Print and shaded views of the part. All mm, measured from the part's lowest x, y and z. A direction names the side the tool comes from. Give positions to 0.01 mm unless a question says otherwise; leave off trailing zeros. Loops run counter-clockwise (first coordinate to the right, second up) from the corner with the lowest first, then second, coordinate; pieces in that order, holes last. Notation, with made-up numbers: M 46.5,81 L 90.5,81 A33 cw 90.5,117 Z; hole C 48.25,39 d6. An arc over 180 degrees is marked long. Answer in a Markdown table with one row per item.
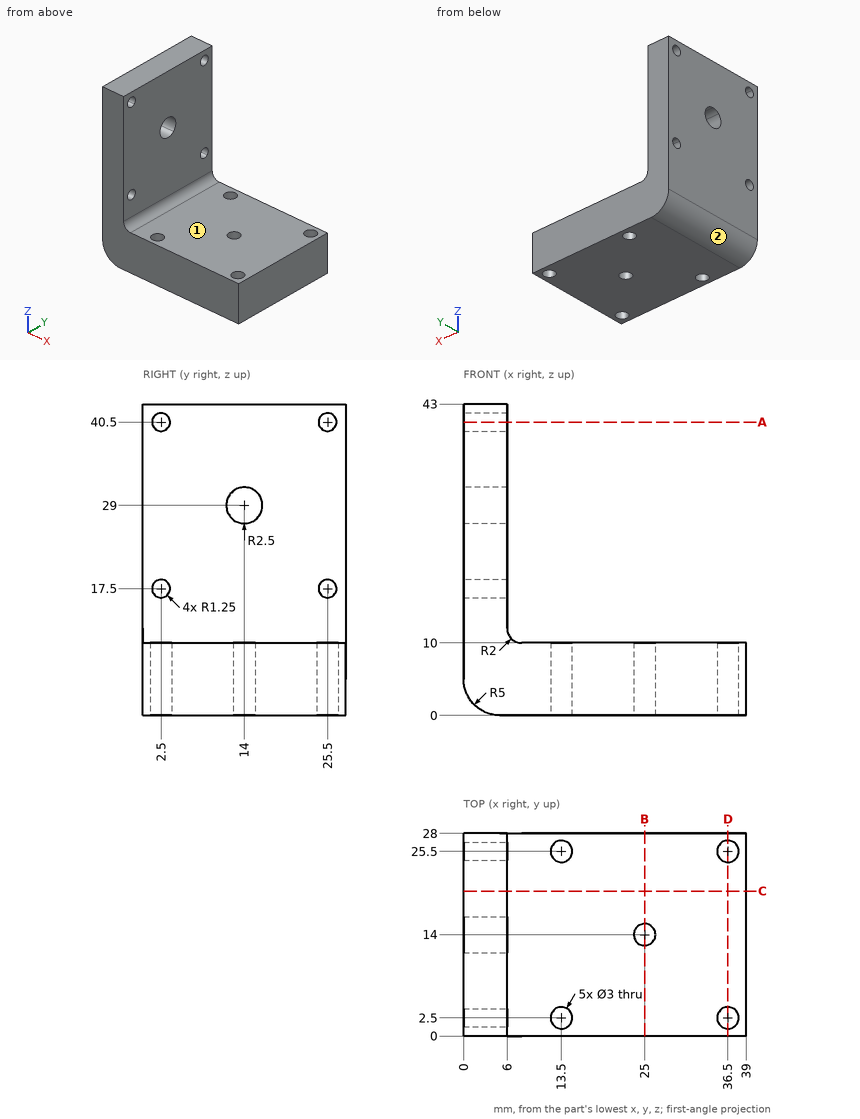
(1) Saw through at D-D, the plane x = 36.5. Give the cut face in (y, z).
Established:
| item | result |
|---|---|
| outline | M 0,0 L 1,0 L 1,10 L 0,10 Z; M 4,0 L 24,0 L 24,10 L 4,10 Z; M 27,0 L 28,0 L 28,10 L 27,10 Z |
(2) Saw through at C-C, the plane y = 20. Give the cut face in (x, z).
Established:
| item | result |
|---|---|
| outline | M 0,5 A5 ccw 5,0 L 39,0 L 39,10 L 8,10 A2 cw 6,12 L 6,43 L 0,43 Z |
(3) Which spindle directions (+Z, -Z, +X, -X, +Y, -Y) get a long thin tool onto all of the face, cutting with end or side? Do the marked faces 1 and 2. Say none if no direction does.
Established:
| item | result |
|---|---|
| face 1 | +Z, +X, +Y, -Y |
| face 2 | -Z, -X, +Y, -Y |
(4) Flat gauge pins, fed straight in: P1, Ø4, axis at x = 36.5, y = 2.5, coming from the -Z side; P2, Ø1.8, axis at x = 13.5, y = 25.5, coming from the +Z side; P3, Ø10, axis at y = 6.5, z = 22, coming from the +X side; P4, Ø3.5, axis at x = 36.5, y = 25.5, coming from the +Z side. Where does each tip first touch, or does it go through?
Established:
| item | result |
|---|---|
| P1 | stops at z = 0 |
| P2 | passes through |
| P3 | stops at x = 6 |
| P4 | stops at z = 10 |
(5) Saw through at B-B, the plane x = 25. Give the cut face in (y, z).
Established:
| item | result |
|---|---|
| outline | M 0,0 L 12.5,0 L 12.5,10 L 0,10 Z; M 15.5,0 L 28,0 L 28,10 L 15.5,10 Z |
(6) Saw through at A-A, the plane z = 40.5. Give the cut face in (x, y), and give its area (3 significant figures).
Established:
| item | result |
|---|---|
| outline | M 0,0 L 6,0 L 6,1.25 L 0,1.25 Z; M 0,3.75 L 6,3.75 L 6,24.25 L 0,24.25 Z; M 0,26.75 L 6,26.75 L 6,28 L 0,28 Z |
| area | 138 mm2 |
(7) Wall check: L1, parallel to Y at x = 13.5, z = 4; L2, parallel to Y at x = 13, z = 9; L3, parallel to Y at x = 25, z = 5. Give the ranges that are in metal, low to high.
Established:
| item | result |
|---|---|
| L1 | y = 0 to 1, 4 to 24, 27 to 28 |
| L2 | y = 0 to 1.09, 3.91 to 24.09, 26.91 to 28 |
| L3 | y = 0 to 12.5, 15.5 to 28 |
